from build123d import *

# Parameters (mm, degrees)
SKETCH1_W           = 25
SKETCH1_H           = 25
BOSS_EXTRUDE1_DEPTH = 4
SKETCH2_W           = 24
SKETCH2_H           = 38
BOSS_EXTRUDE2_DEPTH = 3
SKETCH3_W           = 20
SKETCH3_H           = 2.25
CUT_EXTRUDE1_DEPTH  = 13
SKETCH4_W           = 17
SKETCH4_H           = 3
BOSS_EXTRUDE3_DEPTH = 28
CUT_EXTRUDE2_REACH  = 44.959
SKETCH5_W           = 14
SKETCH5_H           = 17
BOSS_EXTRUDE4_REACH = 48.856
SKETCH6_W           = 1
SKETCH6_H           = 2.25
CUT_EXTRUDE3_REACH  = 49.849
SKETCH7_W           = 2
SKETCH7_H           = 2.25
CUT_EXTRUDE4_REACH  = 44.959
SKETCH9_W           = 21
SKETCH9_H           = 21
SKETCH11_W          = 14
SKETCH11_H          = 17
SKETCH11_W_2        = 13.4
SKETCH11_H_2        = 16.4
BOSS_EXTRUDE5_DEPTH = 1


with BuildPart() as part:
    # Sketch1 → Boss-Extrude1 (new body)
    with BuildSketch(Plane(origin=(0, 0, 0), x_dir=(1, 0, 0), z_dir=(0, 1, 0))):
        Rectangle(SKETCH1_W, SKETCH1_H)
    extrude(amount=BOSS_EXTRUDE1_DEPTH)

    # Sketch2 → Boss-Extrude2 (add)
    with BuildSketch(Plane(origin=(0, 4, 0), x_dir=(1, 0, 0), z_dir=(0, 1, 0))):
        with Locations((0, 6.5)):
            Rectangle(SKETCH2_W, SKETCH2_H)
    extrude(amount=BOSS_EXTRUDE2_DEPTH)

    # Sketch3 → Cut-Extrude1 (cut)
    with BuildSketch(Plane(origin=(0, 0, -25.5), x_dir=(-1, 0, 0), z_dir=(0, 0, -1))):
        with Locations((0, 5.125)):
            Rectangle(SKETCH3_W, SKETCH3_H)
    extrude(amount=-CUT_EXTRUDE1_DEPTH, mode=Mode.SUBTRACT)

    # Sketch4 → Boss-Extrude3 (add)
    with BuildSketch(Plane.XY.offset(12.5)):
        with Locations((0, 5.5)):
            Rectangle(SKETCH4_W, SKETCH4_H)
    extrude(amount=BOSS_EXTRUDE3_DEPTH)

    # Sketch5 → Cut-Extrude2 (cut, up to next)
    with BuildSketch(Plane(origin=(0, 7, 0), x_dir=(1, 0, 0), z_dir=(0, 1, 0)), mode=Mode.PRIVATE) as cut_extrude2_sk1:
        with Locations((0, -30)):
            Rectangle(SKETCH5_W, SKETCH5_H)
    cut_extrude2_tool1 = extrude(cut_extrude2_sk1.sketch, amount=-CUT_EXTRUDE2_REACH, mode=Mode.PRIVATE) & part.part
    add(cut_extrude2_tool1.solids().sort_by_distance((0, 7, 30))[0], mode=Mode.SUBTRACT)

    # Sketch6 → Boss-Extrude4 (add, up to next)
    with BuildSketch(Plane(origin=(-10, 0, 0), x_dir=(0, 0, -1), z_dir=(1, 0, 0)), mode=Mode.PRIVATE) as boss_extrude4_sk1:
        with Locations((25, 5.125)):
            Rectangle(SKETCH6_W, SKETCH6_H)
    boss_extrude4_tool1 = extrude(boss_extrude4_sk1.sketch, amount=BOSS_EXTRUDE4_REACH, mode=Mode.PRIVATE) - part.part
    add(boss_extrude4_tool1.solids().sort_by_distance((-10, 5.125, -25))[0])

    # Sketch7 → Cut-Extrude3 (cut, up to next)
    with BuildSketch(Plane.ZY.offset(12), mode=Mode.PRIVATE) as cut_extrude3_sk1:
        with Locations((-18.5, 5.125)):
            Rectangle(SKETCH7_W, SKETCH7_H)
    cut_extrude3_tool1 = extrude(cut_extrude3_sk1.sketch, amount=-CUT_EXTRUDE3_REACH, mode=Mode.PRIVATE) & part.part
    add(cut_extrude3_tool1.solids().sort_by_distance((-12, 5.125, -18.5))[0], mode=Mode.SUBTRACT)

    # Sketch9 → Cut-Extrude4 (cut, up to next)
    with BuildSketch(Plane.XZ, mode=Mode.PRIVATE) as cut_extrude4_sk1:
        Rectangle(SKETCH9_W, SKETCH9_H)
    cut_extrude4_tool1 = extrude(cut_extrude4_sk1.sketch, amount=-CUT_EXTRUDE4_REACH, mode=Mode.PRIVATE) & part.part
    add(cut_extrude4_tool1.solids().sort_by_distance((0, 0, 0))[0], mode=Mode.SUBTRACT)

    # Sketch11 → Boss-Extrude5 (add)
    with BuildSketch(Plane.XZ.offset(-4)):
        with Locations((0, 30)):
            Rectangle(SKETCH11_W, SKETCH11_H)
        with Locations((0, 30)):
            Rectangle(SKETCH11_W_2, SKETCH11_H_2, mode=Mode.SUBTRACT)
    extrude(amount=-BOSS_EXTRUDE5_DEPTH)


solid = part.part
Model file for the job. Use its own axes, mm. A direction names the side the tool comes from. Give positions to 0.01 mm unless a question says otherwise; leave off trailing zeros. Order: outer loops, then holes, each group sorted by start corner. A loop starts at its lowest first (then second) coordinate and runs counter-clockwise, first axis right, second up. Notation, with made-up numbers: (48.25, 70.5) -> (66.25, 70.5) arc R17 ccw to (66.25, 75.5) -> close; hole circle Ø9 at (11, 3). An arc over 180 degrees is marked (long way). Use CSV: the item, a comma, the result in double quotes.
1. Band-saw the part on C-C, the plane y = 2.75. Give the cut face in (x, z), then the cut area to 3 significant figures.
Outcome:
outline,"(-12.5, -12.5) -> (12.5, -12.5) -> (12.5, 12.5) -> (-12.5, 12.5) -> close; hole (-10.5, -10.5) -> (10.5, -10.5) -> (10.5, 10.5) -> (-10.5, 10.5) -> close"
area,"184 mm²"
2. Band-saw the part on D-D, the plane z = 1.5. Give the cut face in (x, y).
Outcome:
outline,"(-12.5, 0) -> (-10.5, 0) -> (-10.5, 7) -> (-12, 7) -> (-12, 4) -> (-12.5, 4) -> close; (10.5, 0) -> (12.5, 0) -> (12.5, 4) -> (12, 4) -> (12, 7) -> (10.5, 7) -> close"
3. Drop flat-ended pins along their axis: pin 1 (0.9 mm diameter, centred on y = 6, z = 27, fed in from -X); pin 2 (1.1 mm diameter, centred on y = 5, z = -20.5, fed in from -X); pin 3 (0.7 mm diameter, centred on y = 5.5, z = -14, fed in from +X). Give the stop position or say it passes through.
Outcome:
pin 1,"x = -8.5"
pin 2,"x = -12"
pin 3,"x = 12"
4. Mould opens along X. For faces 4 (the flat face through (-12, 5, -6)), 5 (the flat face through (0, 6, 40.5)), 6 (the flat face through (-10, 5, -22)) say: +X half, -X half, draft (parallel to the pull), parting line (faces both ways), or undercut.
Outcome:
face 4,"-X half"
face 5,"draft"
face 6,"undercut"
5. Band-saw the part on B-B, the plane x = 1.5. Give the cut face in (y, z), then the cut area to 3 significant figures.
Outcome:
outline,"(0, -12.5) -> (6.25, -12.5) -> (6.25, -24.5) -> (4, -24.5) -> (4, -25.5) -> (7, -25.5) -> (7, -10.5) -> (0, -10.5) -> close; (0, 10.5) -> (7, 10.5) -> (7, 21.5) -> (5, 21.5) -> (5, 21.8) -> (4, 21.8) -> (4, 12.5) -> (0, 12.5) -> close; (4, 38.2) -> (5, 38.2) -> (5, 38.5) -> (7, 38.5) -> (7, 40.5) -> (4, 40.5) -> close"
area,"73.6 mm²"
6. 3-axis set-ups, long thin cutter, end or side, ignore diameter. For faces 1 (the flat face through (0, 4, 20)), 2 (the flat face through (-7, 6, 30)), 3 (the flat face through (-11, 4, -15)): which of +Z, -Z, +X, -X, +Y, -Y reach the whole face in a straight line?
Outcome:
face 1,"+Z, +X, -X, -Y"
face 2,"+Y"
face 3,"-Z, +X, -X, -Y"
7. Band-saw the part on A-A, the plane z = 33. Give the cut face in (x, y).
Outcome:
outline,"(-8.5, 4) -> (-6.7, 4) -> (-6.7, 5) -> (-7, 5) -> (-7, 7) -> (-8.5, 7) -> close; (6.7, 4) -> (8.5, 4) -> (8.5, 7) -> (7, 7) -> (7, 5) -> (6.7, 5) -> close"
8. Drill centre lines: line 1 along Z through (x, y) = (-7.75, 5.25); line 2 along Z through (x, y) = (-1, 6); line 3 along Z through (x, y) = (-4, 4.75). Where is each one in solid material? Low to high. Write a range as from..to.
Outcome:
line 1,"-25.5..-24.5, -12.5..-10.5, 10.5..40.5"
line 2,"-25.5..-24.5, -12.5..-10.5, 10.5..21.5, 38.5..40.5"
line 3,"-25.5..-24.5, -12.5..-10.5, 10.5..21.8, 38.2..40.5"
